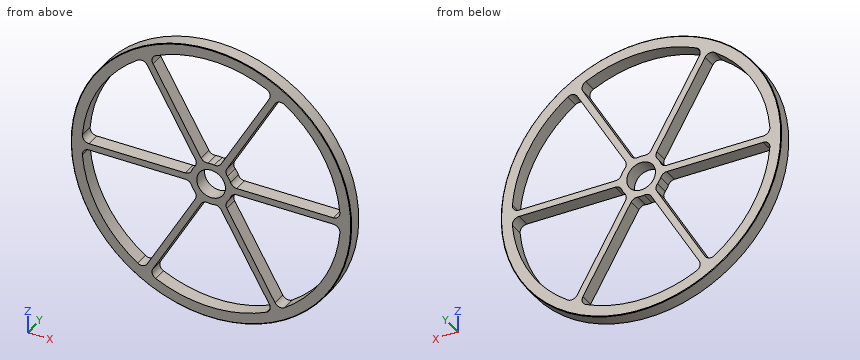
from build123d import *

# Parameters (mm, degrees)
SKETCH1_R           = 63.5
SKETCH1_R_2         = 6.5
BOSS_EXTRUDE3_DEPTH = 6.35
CHAMFER2_SIZE       = 0.25


with BuildPart() as part:
    # Sketch1 → Boss-Extrude3 (new body)
    with BuildSketch(Plane(origin=(0, 0, 0), x_dir=(1, 0, 0), z_dir=(0, 1, 0))):
        with Locations(Location((0, 0, 0), (0, 0, 270))):
            Circle(SKETCH1_R)
        with Locations(Location((0, 0, 0), (0, 0, 270))):
            Circle(SKETCH1_R_2, mode=Mode.SUBTRACT)
        with BuildLine():
            Line((-4.531913789, 10.849504938), (-26.359595266, 48.656158268))
            ThreePointArc((-26.359595266, 48.656158268), (-26.62540639, 51.049550304), (-25.04592549, 52.867301958))
            ThreePointArc((-25.04592549, 52.867301958), (0, 58.5), (25.04592549, 52.867301958))
            ThreePointArc((25.04592549, 52.867301958), (26.62540639, 51.049550304), (26.359595266, 48.656158268))
            Line((26.359595266, 48.656158268), (4.531913789, 10.849504938))
            ThreePointArc((4.531913789, 10.849504938), (3.227737969, 9.642879405), (1.469716559, 9.385623753))
            ThreePointArc((1.469716559, 9.385623753), (0, 9.5), (-1.469716559, 9.385623753))
            ThreePointArc((-1.469716559, 9.385623753), (-3.227737969, 9.642879405), (-4.531913789, 10.849504938))
        make_face(mode=Mode.SUBTRACT)
        with BuildLine():
            Line((7.129990001, 9.349504938), (28.957671478, 47.156158268))
            ThreePointArc((28.957671478, 47.156158268), (30.89750422, 48.583053472), (33.26146378, 48.124058715))
            ThreePointArc((33.26146378, 48.124058715), (50.662486121, 29.25), (58.30738927, 4.743243243))
            ThreePointArc((58.30738927, 4.743243243), (57.52291061, 2.466496832), (55.317266744, 1.5))
            Line((55.317266744, 1.5), (11.66190379, 1.5))
            ThreePointArc((11.66190379, 1.5), (9.964847515, 2.026136625), (8.86304688, 3.42))
            ThreePointArc((8.86304688, 3.42), (8.227241336, 4.75), (7.393330321, 5.965623753))
            ThreePointArc((7.393330321, 5.965623753), (6.737109546, 7.61674278), (7.129990001, 9.349504938))
        make_face(mode=Mode.SUBTRACT)
        with BuildLine():
            Line((11.66190379, -1.5), (55.317266744, -1.5))
            ThreePointArc((55.317266744, -1.5), (57.52291061, -2.466496832), (58.30738927, -4.743243243))
            ThreePointArc((58.30738927, -4.743243243), (50.662486121, -29.25), (33.26146378, -48.124058715))
            ThreePointArc((33.26146378, -48.124058715), (30.89750422, -48.583053472), (28.957671478, -47.156158268))
            Line((28.957671478, -47.156158268), (7.129990001, -9.349504938))
            ThreePointArc((7.129990001, -9.349504938), (6.737109546, -7.61674278), (7.393330321, -5.965623753))
            ThreePointArc((7.393330321, -5.965623753), (8.227241336, -4.75), (8.86304688, -3.42))
            ThreePointArc((8.86304688, -3.42), (9.964847515, -2.026136625), (11.66190379, -1.5))
        make_face(mode=Mode.SUBTRACT)
        with BuildLine():
            Line((4.531913789, -10.849504938), (26.359595266, -48.656158268))
            ThreePointArc((26.359595266, -48.656158268), (26.62540639, -51.049550304), (25.04592549, -52.867301958))
            ThreePointArc((25.04592549, -52.867301958), (0, -58.5), (-25.04592549, -52.867301958))
            ThreePointArc((-25.04592549, -52.867301958), (-26.62540639, -51.049550304), (-26.359595266, -48.656158268))
            Line((-26.359595266, -48.656158268), (-4.531913789, -10.849504938))
            ThreePointArc((-4.531913789, -10.849504938), (-3.227737969, -9.642879405), (-1.469716559, -9.385623753))
            ThreePointArc((-1.469716559, -9.385623753), (0, -9.5), (1.469716559, -9.385623753))
            ThreePointArc((1.469716559, -9.385623753), (3.227737969, -9.642879405), (4.531913789, -10.849504938))
        make_face(mode=Mode.SUBTRACT)
        with BuildLine():
            Line((-7.129990001, -9.349504938), (-28.957671478, -47.156158268))
            ThreePointArc((-28.957671478, -47.156158268), (-30.89750422, -48.583053472), (-33.26146378, -48.124058715))
            ThreePointArc((-33.26146378, -48.124058715), (-50.662486121, -29.25), (-58.30738927, -4.743243243))
            ThreePointArc((-58.30738927, -4.743243243), (-57.52291061, -2.466496832), (-55.317266744, -1.5))
            Line((-55.317266744, -1.5), (-11.66190379, -1.5))
            ThreePointArc((-11.66190379, -1.5), (-9.964847515, -2.026136625), (-8.86304688, -3.42))
            ThreePointArc((-8.86304688, -3.42), (-8.227241336, -4.75), (-7.393330321, -5.965623753))
            ThreePointArc((-7.393330321, -5.965623753), (-6.737109546, -7.61674278), (-7.129990001, -9.349504938))
        make_face(mode=Mode.SUBTRACT)
        with BuildLine():
            Line((-11.66190379, 1.5), (-55.317266744, 1.5))
            ThreePointArc((-55.317266744, 1.5), (-57.52291061, 2.466496832), (-58.30738927, 4.743243243))
            ThreePointArc((-58.30738927, 4.743243243), (-50.662486121, 29.25), (-33.26146378, 48.124058715))
            ThreePointArc((-33.26146378, 48.124058715), (-30.89750422, 48.583053472), (-28.957671478, 47.156158268))
            Line((-28.957671478, 47.156158268), (-7.129990001, 9.349504938))
            ThreePointArc((-7.129990001, 9.349504938), (-6.737109546, 7.61674278), (-7.393330321, 5.965623753))
            ThreePointArc((-7.393330321, 5.965623753), (-8.227241336, 4.75), (-8.86304688, 3.42))
            ThreePointArc((-8.86304688, 3.42), (-9.964847515, 2.026136625), (-11.66190379, 1.5))
        make_face(mode=Mode.SUBTRACT)
    extrude(amount=BOSS_EXTRUDE3_DEPTH)

    # Chamfer2
    chamfer2_edges = [part.edges().sort_by_distance(p)[0] for p in [
        (0, 6.35, -63.5),
        (0, 6.35, -63.5),
        (0, 6.35, -63.5),
        (0, 0, -63.5),
        (0, 0, -63.5),
        (0, 0, -63.5),
        (0, 0, -63.5),
        (0, 6.35, -63.5),
    ]]
    chamfer(chamfer2_edges, length=CHAMFER2_SIZE)


solid = part.part
Work out the finished part from the listing and answer in its coordinate system (mm). Give positions to 0.01 mm unless a question says otherwise; leave off trailing zeros. Order: outer loops, then holes, each group sorted by start corner. A loop starts at its lowest first (then second) coordinate and runs counter-clockwise, first axis right, second up. Notation, with made-up numbers: (-28.5, 7.25) -> (9.5, 7.25) arc R23 cw to (9.5, 31.25) -> close; hole circle Ø11 at (9.25, -29). An arc over 180 degrees is marked (long way). Answer as a JSON object with one key per item and string values. Group by question number.
1. Flat-ended cylindrical pins translate along their axes: pin 1 Ø3 at (x, y) = (-33.5, 2.5) entering from +Z; pin 2 Ø1.5 at (y, z) = (2, 28.5) entering from -X; pin 3 Ø1.5 at (y, z) = (1.5, 38) entering from +X. Find the tip coordinate at first contact, or state that the pin passes through.
2. Section A-A on x = 0 is taken. Determine the outline of the cut face in (y, z).
3. Section C-C on y = 5 is taken. Count the separate pieces of the cut face and the enclosed holes in it, plus the area to 3 significant figures.
4. Consider line 1 along X through (y, z) = (3, 0); line 2 along X through (y, z) = (5, 20) (3 decimals); line 3 along X through (y, z) = (4.75, 37). Determine where each line is inside the solid, lowest interval first. Write a range as [from, to].
5. Section B-B on z = 0 is taken. Determine the outline of the cut face in (x, y), plus the area to 3 significant figures.
Result sheet:
{
 "1": {"pin 1": "stops at z = 54.85", "pin 2": "stops at x = -57.12", "pin 3": "stops at x = 51.43"},
 "2": {"outline": "(0, -63.25) -> (0.25, -63.5) -> (6.1, -63.5) -> (6.35, -63.25) -> (6.35, -58.5) -> (0, -58.5) -> close; (0, -9.5) -> (6.35, -9.5) -> (6.35, -6.5) -> (0, -6.5) -> close; (0, 6.5) -> (6.35, 6.5) -> (6.35, 9.5) -> (0, 9.5) -> close; (0, 58.5) -> (6.35, 58.5) -> (6.35, 63.25) -> (6.1, 63.5) -> (0.25, 63.5) -> (0, 63.25) -> close"},
 "3": {"separate pieces": "1", "enclosed holes": "7", "area": "2,990 mm^2"},
 "4": {"line 1": "x = [-63.5, -6.5], [6.5, 63.5]", "line 2": "x = [-60.268, -54.975], [-13.279, -9.815], [9.815, 13.279], [54.975, 60.268]", "line 3": "x = [-51.61, -45.31], [-23.09, -19.63], [19.63, 23.09], [45.31, 51.61]"},
 "5": {"outline": "(-63.5, 0.25) -> (-63.25, 0) -> (-6.5, 0) -> (-6.5, 6.35) -> (-63.25, 6.35) -> (-63.5, 6.1) -> close; (6.5, 0) -> (63.25, 0) -> (63.5, 0.25) -> (63.5, 6.1) -> (63.25, 6.35) -> (6.5, 6.35) -> close", "area": "724 mm^2"}
}
